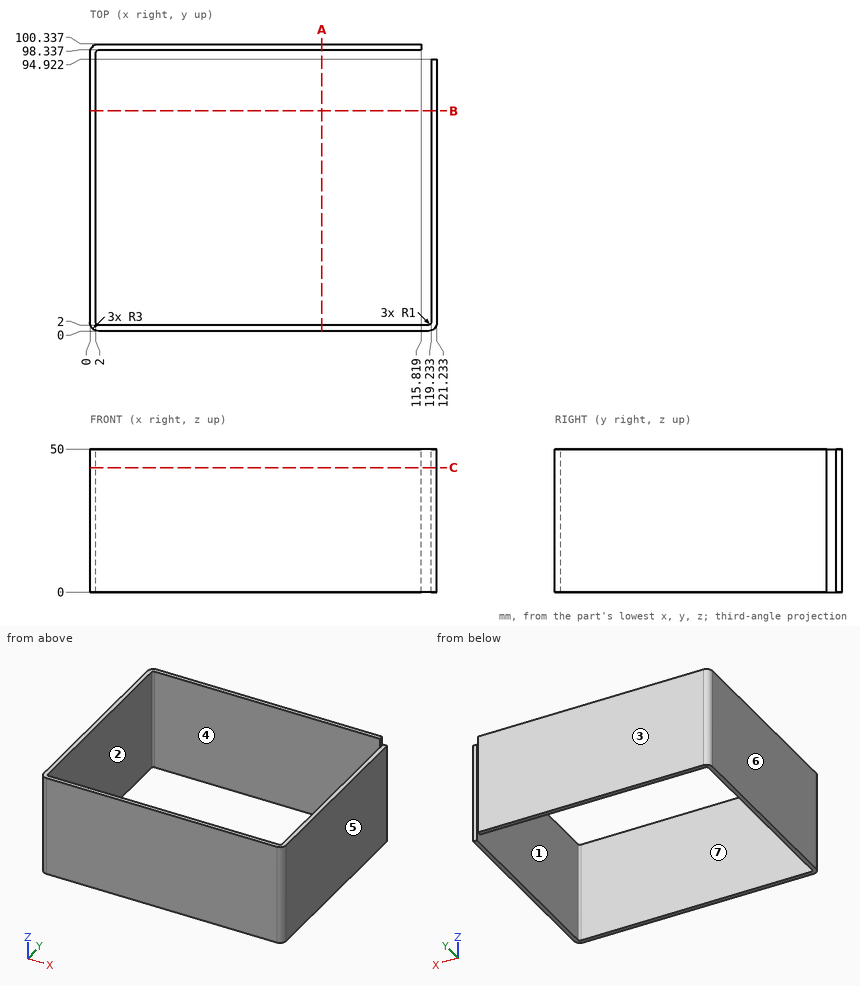
Can you work these out from the drawing? Everything is in mm from the part's minimum corner. A direction names the side the tool comes from. Coordinates: 2 decimals unless noted, no trailing zeros. Loops run counter-clockwise (first coordinate to the right, second up) from the corner with the lowest first, then second, coordinate; pieces in that order, holes last.
1) Which directions (+Z, -Z, +X, -X, +Y, -Y) give clear straight access to the entire face, cutting with the end or side of a thin tool? Please do the marked faces 1, 2 and 3.
Reported:
face 1: +Z, -Z, +Y
face 2: +Z, -Z
face 3: +Z, -Z, +X, -X, +Y
2) Imagine slicing it at A-A (x = 81). List the corners of the cut face in (y, z) for me.
Reported:
outline: (0, 0) - (2, 0) - (2, 50) - (0, 50) - close; (98.34, 0) - (100.34, 0) - (100.34, 50) - (98.34, 50) - close
3) Thinking about a two-plate mould opening in X: for the marked faces 4, 5, 6 and 7, which applies, released by +X, released by -X, zero draft, split by the parting line, or undercut?
Reported:
face 4: zero draft
face 5: released by +X
face 6: released by -X
face 7: undercut
4) Imagine slicing it at B-B (y = 77). List the corners of the cut face in (x, z) for me.
Reported:
outline: (0, 0) - (2, 0) - (2, 50) - (0, 50) - close; (119.23, 0) - (121.23, 0) - (121.23, 50) - (119.23, 50) - close
5) Please list where these lines run through material, in increasing order: line 1 along Y through (x, z) = (90, 44.5); line 2 along X through (y, z) = (23.5, 25.5).
Reported:
line 1: y = 0 to 2, 98.34 to 100.34
line 2: x = 0 to 2, 119.23 to 121.23
6) Will these pins go through, and if not, where does the flat tip stop? pin 1 Ø25 at (x, z) = (68.5, 33.5) entering from -Y; pin 2 Ø1 at (x, z) = (120, 33.5) entering from +Y; pin 3 Ø1.6 at (y, z) = (99, 23) entering from +X.
Reported:
pin 1: stops at y = 0
pin 2: stops at y = 94.92
pin 3: stops at x = 115.82
7) Imagine slicing it at C-C (z = 43.5). List the corners of the cut face in (x, y) for me.
Reported:
outline: (0, 3) arc R3 ccw to (3, 0) - (118.23, 0) arc R3 ccw to (121.23, 3) - (121.23, 94.92) - (119.23, 94.92) - (119.23, 3) arc R1 cw to (118.23, 2) - (3, 2) arc R1 cw to (2, 3) - (2, 97.34) arc R1 cw to (3, 98.34) - (115.82, 98.34) - (115.82, 100.34) - (3, 100.34) arc R3 ccw to (0, 97.34) - close
